from build123d import *

# Parameters (mm, degrees)
F1_DEPTH       = 14
F2_SIZE        = 0.5
F4_D           = 15
F4_CBORE_D     = 19
F4_CBORE_DEPTH = 5
F6_D           = 15
F6_DEPTH       = 17
F6_CBORE_D     = 19
F6_CBORE_DEPTH = 5
F6_TIP         = 4.5064546427
F8_D           = 4.2
F8_DEPTH       = 17
F8_TIP         = 1.2618073
F9_D           = 3
F9_DEPTH       = 8
F9_TIP         = 0.9012909285


with BuildPart() as f1:
    # F0 (on Right) → F1 (new body, symmetric)
    with BuildSketch(Plane.YZ):
        Polygon((0, 20), (0, 0), (22, 0), (22, 52), (-8, 52), (-8, 20), align=None)
    extrude(amount=F1_DEPTH, both=True)

    # F2
    f2_edges = [f1.edges().sort_by_distance(p)[0] for p in [
        (14, 0, 10),
        (14, 11, 0),
        (14, 22, 26),
        (14, 7, 52),
        (14, -8, 36),
        (14, -4, 20),
        (-14, 0, 10),
        (-14, 11, 0),
        (-14, 22, 26),
        (-14, 7, 52),
        (-14, -8, 36),
        (-14, -4, 20),
        (0, 0, 0),
        (0, 22, 0),
        (0, 22, 52),
        (0, -8, 52),
        (0, -8, 20),
    ]]
    chamfer(f2_edges, length=F2_SIZE)

    # F4 (through all)
    with Locations(Plane.XZ.offset(8)):
        with Locations((0, 39)):
            CounterBoreHole(F4_D / 2, F4_CBORE_D / 2, F4_CBORE_DEPTH)

    # F6
    with Locations(Plane(origin=(0, 22, 0), x_dir=(-1, 0, 0), z_dir=(0, 1, 0))):
        with Locations((0, 39)):
            CounterBoreHole(F6_D / 2, F6_CBORE_D / 2, F6_CBORE_DEPTH, depth=F6_DEPTH)
            with Locations((0, 0, -(F6_DEPTH + F6_TIP / 2))):  # 118° drill point
                Cone(0, F6_D / 2, F6_TIP, mode=Mode.SUBTRACT)

    # F8
    with Locations(Plane(origin=(0, 0, 0), x_dir=(1, 0, 0), z_dir=(0, 0, -1))):
        with Locations((0, -11)):
            Hole(F8_D / 2, depth=F8_DEPTH)
            with Locations((0, 0, -(F8_DEPTH + F8_TIP / 2))):  # 118° drill point
                Cone(0, F8_D / 2, F8_TIP, mode=Mode.SUBTRACT)

    # F9
    with Locations(Plane(origin=(0, 0, 0), x_dir=(1, 0, 0), z_dir=(0, 0, -1))):
        with Locations((-9, -5), (9, -17)):
            Hole(F9_D / 2, depth=F9_DEPTH)
            with Locations((0, 0, -(F9_DEPTH + F9_TIP / 2))):  # 118° drill point
                Cone(0, F9_D / 2, F9_TIP, mode=Mode.SUBTRACT)


solid = f1.part
For this review, take the finished solid that the model builds, in its own axes (mm). A direction names the side the tool comes from. Round coordinates to 2 decimals unless told otherwise and drop trailing zeros. Loops run counter-clockwise (first coordinate to the right, second up) from the corner with the lowest first, then second, coordinate; pieces in that order, holes last. Notation, with made-up numbers: (14.25, 77.5) - (68.25, 77.5) arc R17 ccw to (68.25, 83.5) - close; hole circle Ø6 at (3.5, 15). An arc over 180 degrees is marked (long way). One line per item, written item: value. Start each with the question number.
Item 1: Take a section at C-C (z = 39). Give the boundary of the cut face in (x, y).
Item 2: Take a section at B-B (x = 11.5). Give the boundary of the cut face in (y, z).
Item 3: Clearance check with flat-ended pins moving along their axes: pin 1 Ø6.5 at (x, y) = (0, 11) entering from -Z; pin 2 Ø8.5 at (x, y) = (-6.5, -4) entering from -Z; pin 3 Ø6 at (x, y) = (10.5, -4) entering from -Z; pin 4 Ø15.5 at (x, z) = (5.5, 10.5) entering from -Y. State where each tip first meets the part, or that it passes through.
Item 4: For faces 1 (the flat face through (0, -4, 20)), 2 (the cylindrical face through (-1.24, -5.54, 48.42)), 3 (the cylindrical face through (10.11, 15.99, 4.06)), list the 3-axis set-ups (+Z, -Z, +X, -X, +Y, -Y) from which the entire face can be reached by the end or side of a thin tool; tool diameter is ignored.
Item 5: Take a section at D-D (z = 15). Give the boundary of the cut face in (x, y), plus the area to 3 significant figures.
Item 6: The part is to be moulded in two halves that separate along X. For faces 4 (the cylindrical face through (-7.89, 3.99, 4.06)), 5 (the flat face through (-1, 17, 47)), 6 (the flat face through (0, 0, 10)), 7 (the flat face through (-14, 7, 26)), say which applies: +X half, -X half, draft (parallel to the pull), parting line (faces both ways), or undercut.
Item 7: For L1, parallel to Z at x = 0, y = 18.35; L2, parallel to Y at x = 9, z = 5.5; L3, parallel to X at y = 17, z = 6.5, list the stretches that pass through material, from the lowest coordinate up.
Item 8: Take a section at A-A (y = -4.5). Give the boundary of the cut face in (x, z).
Answer below:
1. outline: (-14, -7.5) - (-13.5, -8) - (-9.5, -8) - (-9.5, -3) - (-7.5, -3) - (-7.5, 17) - (-9.5, 17) - (-9.5, 22) - (-13.5, 22) - (-14, 21.5) - close; (7.5, -3) - (9.5, -3) - (9.5, -8) - (13.5, -8) - (14, -7.5) - (14, 21.5) - (13.5, 22) - (9.5, 22) - (9.5, 17) - (7.5, 17) - close
2. outline: (-8, 20.5) - (-7.5, 20) - (0, 20) - (0, 0.5) - (0.5, 0) - (21.5, 0) - (22, 0.5) - (22, 51.5) - (21.5, 52) - (-7.5, 52) - (-8, 51.5) - close
3. pin 1: stops at z = 0
3. pin 2: stops at z = 0.25
3. pin 3: stops at z = 20
3. pin 4: stops at y = 0
4. face 1: -Z, +X, -X, -Y
4. face 2: -Y
4. face 3: -Z
5. outline: (-14, 0.5) - (-13.5, 0) - (13.5, 0) - (14, 0.5) - (14, 21.5) - (13.5, 22) - (-13.5, 22) - (-14, 21.5) - close; hole circle Ø4.2 at (0, 11)
5. area: 602 mm2
6. face 4: undercut
6. face 5: undercut
6. face 6: draft
6. face 7: -X half
7. L1: z = 0 to 29.5, 48.5 to 52
7. L2: y = 0 to 15.5, 18.5 to 22
7. L3: x = -14 to 7.5, 10.5 to 14
8. outline: (-14, 20.5) - (-13.5, 20) - (13.5, 20) - (14, 20.5) - (14, 51.5) - (13.5, 52) - (-13.5, 52) - (-14, 51.5) - close; hole circle Ø19 at (0, 39)
